Autodesk Inventor part; units mm, degrees
ref_plane "YZ Plane" through (0, 0, 0) normal (1, 0, 0) x (0, 1, 0)
ref_plane "XZ Plane" through (0, 0, 0) normal (0, 1, 0) x (-1, 0, 0)
ref_plane "XY Plane" through (0, 0, 0) normal (0, 0, 1) x (1, 0, 0)
sketch "Sketch1" plane through (0, 0, 0) normal (0, 1, 0) x (-1, 0, 0)
  circle A0 centre (0, 0) radius 3.75
  circle A1 centre (0, 0) radius 6
  circle A2 centre (-45, 0) radius 2
  circle A3 centre (-45, 0) radius 6
  line L0 (0, 6) -> (-45, 6)
  line L1 (0, -6) -> (-45, -6)
  dimension "d0" = 7.5
  dimension "d1" = 12
  dimension "d2" = 4
  dimension "d3" = 45
  dimension "d4" = 12
extrude "Extrusion2" add sketch "Sketch1" along normal blind 4
sketch "Sketch2" plane through (0, 4, 0) normal (0, 1, 0) x (1, 0, 0)
  arc A0 (14.3366, -2.2384) -> (14.3439, 2.2376) centre (14.108, 0) ccw
  circle A1 centre (0, 0) radius 3.75
  arc A2 (0.7821, 3.6675) -> (2.5223, -2.775) centre (0, 0) ccw
  line L0 (0.7821, 3.6675) -> (14.3439, 2.2376)
  line L1 (14.3366, -2.2384) -> (0, -3.75)
  point P0 (2.5223, 2.775)
  dimension "d9" = 14.108
  dimension "d10" = 4.5
  dimension "d11" = 2.775
  dimension "d12" = 2.5223
  dimension "d13" = 5.55
extrude "Extrusion3" cut sketch "Sketch2" against normal blind 2 contours L1 A1 L0 A0
properties part number "Stewart_ServoArm"
The model under review builds one solid part; all positions refer to its coordinate system, in mm. A direction names the side the tool comes from. Round coordinates to 2 decimals unless told otherwise and drop trailing zeros. Order: outer loops, then holes, each group sorted by start corner. A loop starts at its lowest first (then second) coordinate and runs counter-clockwise, first axis right, second up. Notation, with made-up numbers: (74.25, -12.5) - (94.25, -12.5) arc R35 ccw to (94.25, 25.5) - close; hole circle Ø5 at (31, 59). An arc over 180 degrees is marked (long way). Use one line per item in the form item = value.
Q1. To check wall thickness, follow line 1 (Z direction, x = 45, y = 1.05); line 2 (X direction, y = 3.55, z = 1.75); line 3 (X direction, y = 0.45, z = -0.5). State the ranges of each line that lie inside material, in increasing order.
Response values:
line_1 = -6 to -2, 2 to 6
line_2 = -5.74 to -3.32, 15.52 to 44.03, 45.97 to 50.74
line_3 = -5.98 to -3.72, 3.72 to 43.06, 46.94 to 50.98
Q2. Add section B-B on x = 46. Give the boundary of the cut face in (y, z).
Response values:
outline = (0, -5.92) - (4, -5.92) - (4, -1.73) - (0, -1.73) - close; (0, 1.73) - (4, 1.73) - (4, 5.92) - (0, 5.92) - close
Q3. Add section C-C on x = 15. Give the boundary of the cut face in (y, z), then the cut area to 3 significant figures.
Response values:
outline = (0, -6) - (4, -6) - (4, -2.07) - (2, -2.07) - (2, 2.07) - (4, 2.07) - (4, 6) - (0, 6) - close
area = 39.7 mm^2
Q4. Tool access review of faces 4 (the cylindrical face through (16.357, 3.014, 0.05)), 5 (the cylindrical face through (-3.577, 1.528, -1.126)): name each direction out of +Z, -Z, +X, -X, +Y, -Y from which nothing blocks a thin tool from reaching the whole face with its end or side.
Response values:
face_4 = +Y
face_5 = +Y, -Y
Q5. Mouldability with a two-part tool opening along Z and no side actions: class faces 1 (the cylindrical face through (51, 2, 0)), 2 (the flat face through (7.654, 3.014, 2.943)), 3 (the flat face through (29, 4, 0)) as pulls with the +Z half, pulls with the -Z half, needs draft (parallel to the pull), parting line crosses it, or undercut.
Response values:
face_1 = parting line crosses it
face_2 = undercut
face_3 = needs draft
Q6. Clearance check with flat-ended pins moving along their axes: P1, Ø3.5, axis at x = 5, z = -1.5, coming from the +Y side; P2, Ø3, axis at x = 45, z = 0, coming from the -Y side. State where each tip first meets the part, or that it passes through.
Response values:
P1 = 4
P2 = through
Q7. Add section A-A on y = 3.3. Give the boundary of the cut face in (x, z).
Response values:
outline = (0, -6) - (45, -6) arc R6 ccw to (45, 6) - (0, 6) arc R6 ccw to start; hole (0.78, -3.67) - (14.34, -2.24) arc R2.25 ccw to (14.34, 2.24) - (0.78, 3.67) arc R3.75 ccw (long way) to start; hole circle Ø4 at (45, 0)
